For this review, use the dimensioned drawing (mm, ordinates from the lowest corner) and the shaded views. A direction names the side the tool comes from. Give positions to 0.01 mm unless a question says otherwise; leave off trailing zeros. Order: outer loops, then holes, each group sorted by start corner. A loop starts at its lowest first (then second) coordinate and runs counter-clockwise, first axis right, second up. Notation, with made-up numbers: (35, -1.5) -> (48, -1.5) arc R20 cw to (48, 2.5) -> close; hole circle Ø8 at (7, -37.75). An arc over 180 degrees is marked (long way). Answer as a JSON object with one key per item and string values. Group by question number.
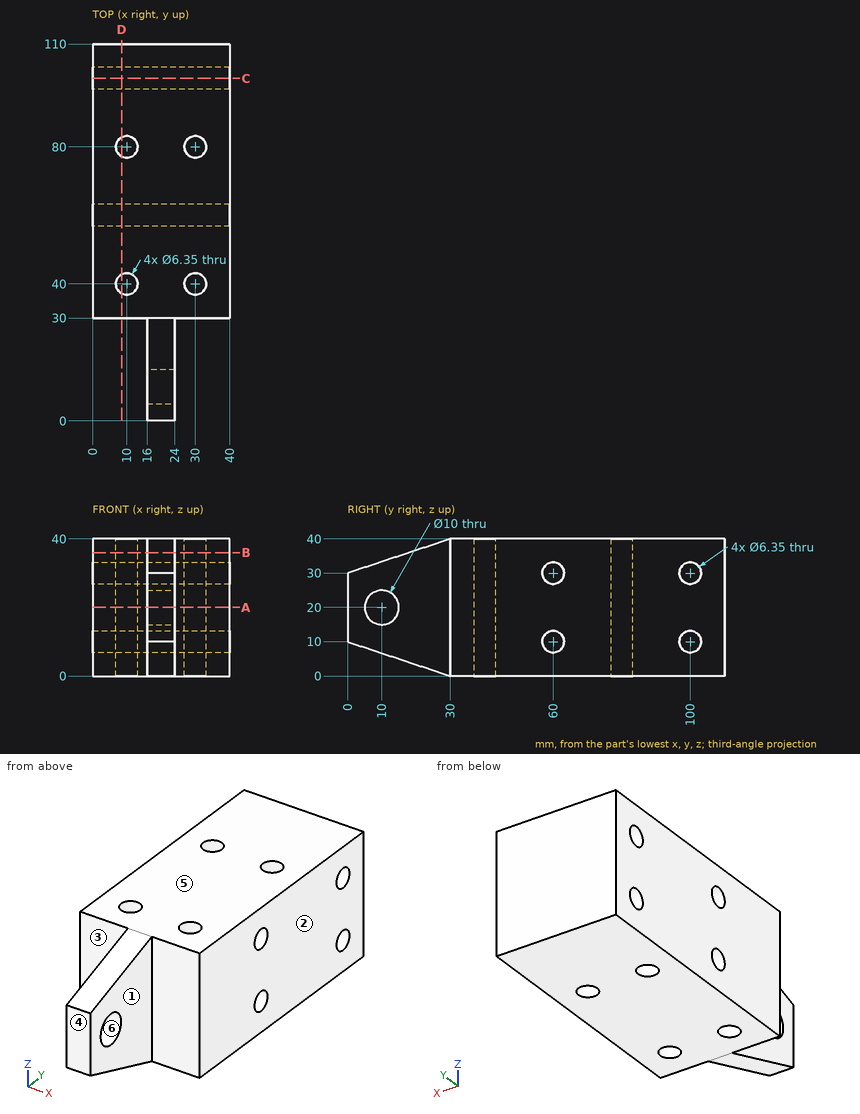
1. Machinability: for the marked faces 1, 2 and 3, which of the approach directions +Z, -Z, +X, -X, +Y, -Y give a long, thin tool a straight path to every point of the face, cutting with its end or side? Answer none if there is none.
2. For pin 1 (13 mm diameter, centred on x = 7.5, z = 30, fed in from -Y); pin 2 (5 mm diameter, centred on x = 30, y = 40, fed in from +Z), all flat-tipped, find the tip position at first contact; note any pin that passes through.
3. Take a section at B-B on z = 36. Give the boundary of the cut face in (x, y) (3 decimals), plus the area to 3 significant figures.
4. Take a section at D-D on x = 8.5. Give the boundary of the cut face in (y, z) (3 decimals), plus the area to 3 significant figures.
5. For probe 1 along Z at (x, y) = (17, 60) (3 decimals); probe 2 along Y at (x, z) = (10, 19) (3 decimals), list the stretches that pass through material, from the lowest coordinate up. Write a range as [from, to].
6. Take a section at C-C on y = 100. Give the boundary of the cut face in (x, z) (3 decimals), plus the area to 3 significant figures.
7. Draft analysis for pull direction Y (two halves, no side actions). For the marked faces 4, 5 and 6, state which applies: pulls with the +Y half, pulls with the -Y half, needs draft (parallel to the pull), parting line crosses it, or undercut.
8. Take a section at A-A on z = 20. Give the boundary of the cut face in (x, y) (3 decimals), plus the area to 3 significant figures.
Checks:
{
 "1": {"face 1": "+Z, -Z, +X, -Y", "face 2": "+Z, -Z, +X, +Y, -Y", "face 3": "+Z, -Z, -X, -Y"},
 "2": {"pin 1": "stops at y = 30", "pin 2": "passes through"},
 "3": {"outline": "(0, 30) -> (16, 30) -> (16, 18) -> (24, 18) -> (24, 30) -> (40, 30) -> (40, 110) -> (0, 110) -> close; hole circle Ø6.35 at (10, 40); hole circle Ø6.35 at (10, 80); hole circle Ø6.35 at (30, 40); hole circle Ø6.35 at (30, 80)", "area": "3,170 mm2"},
 "4": {"outline": "(30, 0) -> (37.202, 0) -> (37.202, 40) -> (30, 40) -> close; (42.798, 0) -> (77.202, 0) -> (77.202, 40) -> (42.798, 40) -> close; (82.798, 0) -> (110, 0) -> (110, 40) -> (82.798, 40) -> close; hole circle Ø6.35 at (60, 10); hole circle Ø6.35 at (60, 30); hole circle Ø6.35 at (100, 10); hole circle Ø6.35 at (100, 30)", "area": "2,630 mm2"},
 "5": {"probe 1": "z = [0, 6.825], [13.175, 26.825], [33.175, 40]", "probe 2": "y = [30, 36.825], [43.175, 76.825], [83.175, 110]"},
 "6": {"outline": "(0, 0) -> (40, 0) -> (40, 6.825) -> (0, 6.825) -> close; (0, 13.175) -> (40, 13.175) -> (40, 26.825) -> (0, 26.825) -> close; (0, 33.175) -> (40, 33.175) -> (40, 40) -> (0, 40) -> close", "area": "1,090 mm2"},
 "7": {"face 4": "pulls with the -Y half", "face 5": "needs draft", "face 6": "undercut"},
 "8": {"outline": "(0, 30) -> (16, 30) -> (16, 15) -> (24, 15) -> (24, 30) -> (40, 30) -> (40, 110) -> (0, 110) -> close; (16, 0) -> (24, 0) -> (24, 5) -> (16, 5) -> close; hole circle Ø6.35 at (10, 40); hole circle Ø6.35 at (10, 80); hole circle Ø6.35 at (30, 40); hole circle Ø6.35 at (30, 80)", "area": "3,230 mm2"}
}
